from build123d import *

# Parameters (mm, degrees)
F0_R     = 20
F0_R_2   = 15
F1_DEPTH = 126
F2_R     = 20
F3_DEPTH = 2
F4_R     = 6.692615
F4_R_2   = 3.950799
F5_DEPTH = 15


with BuildPart() as f1:
    # F0 (on Top) → F1 (new body)
    with BuildSketch(Plane.XY):
        Circle(F0_R)
        Circle(F0_R_2, mode=Mode.SUBTRACT)
    extrude(amount=F1_DEPTH)

    # F2 (on face) → F3 (join)
    with BuildSketch(Plane(origin=(0, 0, 0), x_dir=(1, 0, 0), z_dir=(0, 0, -1))):
        Circle(F2_R)
    extrude(amount=F3_DEPTH)

    # F4 (on face) → F5 (join)
    with BuildSketch(Plane(origin=(0, 0, -2), x_dir=(1, 0, 0), z_dir=(0, 0, -1))):
        Circle(F4_R)
        Circle(F4_R_2, mode=Mode.SUBTRACT)
    extrude(amount=F5_DEPTH)


solid = f1.part
Source: CAD feature listing. Evaluate the final solid. Frame: model axes, mm. A direction names the side the tool comes from. Coordinates: 2 decimals unless noted, no trailing zeros. Write each loop counter-clockwise with the first axis right and the second up, starting at its lowest first coordinate (ties: lowest second). Pieces come first, ordered by that corner, then holes. Notation, with made-up numbers: M 18.5,36.25 L 28.5,36.25 A28 ccw 28.5,75.25 Z; hole C -19.5,24.5 d9. An arc over 180 degrees is marked long. Use a Markdown table: item, result.
1) Section D-D, the plane z = 114. Output: boundary loops of the cut face in (x, y).
Conclusion:
| item | result |
|---|---|
| outline | C 0,0 d40; hole C 0,0 d30 |
2) Ray query, L1, parallel to X at y = 0, z = -10.75; L2, parallel to Z at x = 8, y = 15. Return the intervals inside material, ascending.
Conclusion:
| item | result |
|---|---|
| L1 | x = -6.69 to -3.95, 3.95 to 6.69 |
| L2 | z = -2 to 126 |
3) Section C-C, the plane z = -6. Output: boundary loops of the cut face in (x, y).
Conclusion:
| item | result |
|---|---|
| outline | C 0,0 d13.39; hole C 0,0 d7.9 |
4) Mould query, pull axis Y, two halves, no side actions, for faces 1 (the cylindrical face through (-3.947, -0.174, -9.395)), 2 (the cylindrical face through (-1.451, 6.533, -9.395)), 3 (the flat face through (0, 9, -2)). Classes: pulls with the +Y half, pulls with the -Y half, needs draft (parallel to the pull), parting line crosses it, or undercut.
Conclusion:
| item | result |
|---|---|
| face 1 | undercut |
| face 2 | parting line crosses it |
| face 3 | needs draft |
5) First-contact query: pin 1 Ø20 at (x, y) = (-6.5, -6.5) entering from -Z; pin 2 Ø1.5 at (y, z) = (-2.5, 1.5) entering from +X; pin 3 Ø4 at (x, y) = (1, 3) entering from +Z; pin 4 Ø1 at (y, z) = (-7, 80.5) entering from -X. Flat tips, straight axial feed; report the tip coordinate or a pass-through.
Conclusion:
| item | result |
|---|---|
| pin 1 | stops at z = -17 |
| pin 2 | stops at x = 19.92 |
| pin 3 | stops at z = 0 |
| pin 4 | stops at x = -18.91 |
6) Section A-A, the plane y = 0. Output: boundary loops of the cut face in (x, z).
Conclusion:
| item | result |
|---|---|
| outline | M -20,-2 L -6.69,-2 L -6.69,-17 L -3.95,-17 L -3.95,-2 L 3.95,-2 L 3.95,-17 L 6.69,-17 L 6.69,-2 L 20,-2 L 20,126 L 15,126 L 15,0 L -15,0 L -15,126 L -20,126 Z |
7) Reachability of faces 4 (the flat face through (3, 3, -17)), 5 (the flat face through (0, 0, -2)), 6 (the flat face through (0, 0, 0)) from +Z, -Z, +X, -X, +Y, -Y: full face, straight path, thin tool, end or side. Return the list, or none.
Conclusion:
| item | result |
|---|---|
| face 4 | -Z, +X, -X, +Y, -Y |
| face 5 | -Z |
| face 6 | +Z |
